Autodesk Inventor part; units mm, degrees
ref_plane "YZ Plane" through (0, 0, 0) normal (1, 0, 0) x (0, 1, 0)
ref_plane "XZ Plane" through (0, 0, 0) normal (0, 1, 0) x (-1, 0, 0)
ref_plane "XY Plane" through (0, 0, 0) normal (0, 0, 1) x (1, 0, 0)
sketch "Sketch1" plane through (0, 0, 0) normal (0, 1, 0) x (-1, 0, 0)
  line L0 (-0.4654, 17.4069) -> (54.4394, 17.4069)
  line L1 (69.5346, 3.0665) -> (69.5346, -22.5931)
  arc A0 (69.5346, 3.0665) -> (54.4394, 17.4069) centre (53.1439, 0.9282) ccw
  point P0 (0, 0)
  dimension "d0" = 70
  dimension "d1" = 40
sketch "Sketch2" plane through (0, 0, 0) normal (1, 0, 0) x (0, 1, 0)
  line L0 (-5, 15.4069) -> (5, 15.4069)
  line L1 (5, 15.4069) -> (5, 19.4069)
  line L2 (5, 19.4069) -> (-5, 19.4069)
  line L3 (-5, 19.4069) -> (-5, 15.4069)
  point P0 (0, 0)
  point P1 (0, 17.4069)
  dimension "d2" = 10
  dimension "d3" = 5
  dimension "d4" = 4
  dimension "d5" = 2
sweep "Sweep1" add profiles "Sketch2" path "Sketch1"
sketch "Sketch3" plane through (0.4654, -5, 19.4069) normal (0, 0, 1) x (1, 0, 0)
  arc A0 (-3.5, 3.5) -> (-3.5, 6.5) centre (-3.5, 5) ccw
  arc A1 (-33.5, 6.5) -> (-33.5, 3.5) centre (-33.5, 5) ccw
  line L0 (-3.5, 3.5) -> (-33.5, 3.5)
  line L1 (-3.5, 6.5) -> (-33.5, 6.5)
  line L2 (0, 10) -> (-54.9833, 10)
  line L3 (0, 10) -> (0, 0)
  point P0 (-0.4654, 5)
  dimension "d8" = 3
  dimension "d9" = 3
  dimension "d10" = 5
  dimension "d11" = 3.5
  dimension "d12" = 30
extrude "Extrusion1" cut sketch "Sketch3" against normal through all
sketch "Sketch4" plane through (-71.5346, -5, -22.5931) normal (-1, 0, 0) x (0, 0, 1)
  line L0 (0, 10) -> (25.7895, 10)
  line L1 (0, 0) -> (0, 10)
  line L2 (0, 0) -> (25.7895, 0)
  line L3 (25.7895, 10) -> (25.7895, 0)
  line L4 (0, 0) -> (10, 0)
  line L5 (10, 0) -> (10, -3)
  line L6 (10, -3) -> (0, -3)
  line L7 (0, -3) -> (0, 0)
  circle A0 centre (3, 7) radius 1.5
  circle A1 centre (7, 0) radius 1.5
  point P0 (22.5931, 5)
  dimension "d15" = 3
  dimension "d16" = 10
  dimension "d17" = 3
  dimension "d18" = 3
  dimension "d19" = 3
  dimension "d20" = 3
  dimension "d21" = 3
  dimension "d22" = 3
extrude "Extrusion2" add sketch "Sketch4" against normal up to surface (4 mm away) contours L2 A1 L5 L6 L7 | L2 A1 picked at (6.8227, -0.4675)
extrude "Extrusion3" cut sketch "Sketch4" against normal through all contours A1 L2 | L2 A1 | A0
sketch "Sketch5" plane through (-67.5346, 5, -22.5931) normal (0, 0, -1) x (-1, 0, 0)
  line L0 (0, 0) -> (0, -13)
  line L1 (4, -13) -> (0, -13)
  line L2 (4, 0) -> (4, -13)
  line L3 (4, 0) -> (0, 0)
  circle A0 centre (5, -6.5) radius 2
  point P0 (-67.5346, -5)
  dimension "d27" = 4
  dimension "d28" = 6.5
  dimension "d31" = 1
extrude "Extrusion4" cut sketch "Sketch5" against normal through all contours A0 L2 | L2 A0
properties part number "eye_cam_arm"
The model under review builds one solid part; all positions refer to its coordinate system, in mm. A direction names the side the tool comes from. Give positions to 0.01 mm unless a question says otherwise; leave off trailing zeros. Write each loop counter-clockwise with the first axis right and the second up, starting at its lowest first coordinate (ties: lowest second). Pieces come first, ordered by that corner, then holes.
(1) Tool access review of faces 5 (the flat face through (-70, -8, -18)), 6 (the flat face through (-18, 1.5, 17)), 7 (the flat face through (-70, -6, -12.593)), 8 (the flat face through (-27, 2, 15.407)): name each direction out of +Z, -Z, +X, -X, +Y, -Y from which nothing blocks a thin tool from reaching the whole face with its end or side.
(2) Consider section C-C, the plane x = -50.5. Give the boundary of the cut face in (y, z), and give its area (3 significant figures).
(3) For P1, Ø2.5, axis at y = 2, z = -19.59, coming from the +X side; P2, Ø8, axis at x = -38.5, z = 13, coming from the -Y side; P3, Ø3.5, axis at x = -70.5, y = -7, coming from the +Z side; P4, Ø5, axis at x = -47, y = 2.5, coming from the -Z side, all flat-tipped, find the tip position at first contact; note any pin that passes through.
(4) To check wall thickness, follow L1, parallel to Z at x = -44, y = -1; L2, parallel to X at y = -7.5, z = -17; L3, parallel to X at y = 1.25, z = 4.5. State the ranges of each line that lie inside material, in increasing order.
(5) The part is to be moulded in two halves that separate along X. For faces 1 (the flat face through (-67.535, 0, -10)), 2 (the cylindrical face through (-34.534, 0.033, 17.435)), 3 (the flat face through (-18, -1.5, 17)), 4 (the flat face through (-27, -2, 19.407)), say which applies: released by +X, released by -X, zero draft, split by the parting line, or undercut.
(6) Consider section B-B, the plane z = -3.5. Give the boundary of the cut face in (x, y).
(7) Consider section A-A, the plane x = -23. Give the boundary of the cut face in (y, z), and give its area (3 significant figures).
Returned:
1. face 5: +Z, -Z, +X, -X, -Y
1. face 6: +Z, -Z
1. face 7: +Z, +X, -X, -Y
1. face 8: -Z, +X, +Y, -Y
2. outline: (-5, 15.41) - (5, 15.41) - (5, 19.41) - (-5, 19.41) - close
2. area: 40.0 mm2
3. P1: passes through
3. P2: stops at y = -5
3. P3: stops at z = -12.59
3. P4: stops at z = 15.41
4. L1: z = 15.41 to 19.41
4. L2: x = -71.53 to -67.53
4. L3: x = -71.33 to -67.23
5. face 1: released by +X
5. face 2: undercut
5. face 3: undercut
5. face 4: zero draft
6. outline: (-71.53, -5) - (-67.53, -5) - (-67.53, 5) - (-71.53, 5) - (-71.53, 0.23) arc R2 cw to (-71.53, -3.23) - close
7. outline: (-5, 15.41) - (-1.5, 15.41) - (-1.5, 19.41) - (-5, 19.41) - close; (1.5, 15.41) - (5, 15.41) - (5, 19.41) - (1.5, 19.41) - close
7. area: 28.0 mm2
